from build123d import *

# Parameters (mm, degrees)
SKETCH1_W           = 60
SKETCH1_H           = 90
BOSS_EXTRUDE1_DEPTH = 3
SKETCH2_W           = 10
SKETCH2_H           = 3
SKETCH2_W_2         = 3
SKETCH2_H_2         = 10
SKETCH2_W_3         = 20
CUT_EXTRUDE2_DEPTH  = 3
SKETCH3_W           = 80
SKETCH3_H           = 120
BOSS_EXTRUDE2_DEPTH = 3
FILLET1_R           = 10
FILLET2_R           = 10
SKETCH4_R           = 1.7
CUT_EXTRUDE3_DEPTH  = 3
SKETCH5_R           = 11
CUT_EXTRUDE4_DEPTH  = 3
SKETCH6_W           = 20
SKETCH6_H           = 65
BOSS_EXTRUDE3_DEPTH = 3
FILLET3_R           = 10
SKETCH7_R           = 4
CUT_EXTRUDE5_DEPTH  = 3


with BuildPart() as part:
    # Sketch1 → Boss-Extrude1 (new body)
    with BuildSketch(Plane(origin=(0, 0, 0), x_dir=(1, 0, 0), z_dir=(0, 1, 0))):
        Rectangle(SKETCH1_W, SKETCH1_H)
    extrude(amount=BOSS_EXTRUDE1_DEPTH)

    # Sketch2 → Cut-Extrude2 (cut)
    with BuildSketch(Plane(origin=(0, 3, 0), x_dir=(1, 0, 0), z_dir=(0, 1, 0))):
        with Locations((25, 16.5)):
            Rectangle(SKETCH2_W, SKETCH2_H)
        with Locations((-28.5, 30)):
            Rectangle(SKETCH2_W_2, SKETCH2_H_2)
        with Locations((-25, 16.5)):
            Rectangle(SKETCH2_W, SKETCH2_H)
        with Locations((0, 16.5)):
            Rectangle(SKETCH2_W_3, SKETCH2_H)
        with Locations((28.5, 30)):
            Rectangle(SKETCH2_W_2, SKETCH2_H_2)
    extrude(amount=-CUT_EXTRUDE2_DEPTH, mode=Mode.SUBTRACT)

    # Sketch3 → Boss-Extrude2 (add)
    with BuildSketch(Plane(origin=(0, 3, 0), x_dir=(1, 0, 0), z_dir=(0, 1, 0))):
        Rectangle(SKETCH3_W, SKETCH3_H)
        Polygon((-30, 18), (-30, -45), (30, -45), (30, 18), (30, 25), (30, 45), (-30, 45), (-30, 35), align=None, mode=Mode.SUBTRACT)
    extrude(amount=-BOSS_EXTRUDE2_DEPTH)

    # Fillet1
    fillet1_edges = [part.edges().sort_by_distance(p)[0] for p in [
        (-40, 1.5, 60),
        (40, 1.5, 60),
    ]]
    fillet(fillet1_edges, radius=FILLET1_R)

    # Fillet2
    fillet2_edges = [part.edges().sort_by_distance(p)[0] for p in [
        (-40, 1.5, -60),
        (40, 1.5, -60),
    ]]
    fillet(fillet2_edges, radius=FILLET2_R)

    # Sketch4 → Cut-Extrude3 (cut)
    with BuildSketch(Plane(origin=(0, 3, 0), x_dir=(1, 0, 0), z_dir=(0, 1, 0))):
        with Locations(Location((15.5, -9.5, 0), (0, 0, 270))):
            Circle(SKETCH4_R)
        with Locations(Location((15.5, -40.5, 0), (0, 0, 270))):
            Circle(SKETCH4_R)
        with Locations(Location((-15.5, -40.5, 0), (0, 0, 270))):
            Circle(SKETCH4_R)
        with Locations(Location((-15.5, -9.5, 0), (0, 0, 270))):
            Circle(SKETCH4_R)
    extrude(amount=-CUT_EXTRUDE3_DEPTH, mode=Mode.SUBTRACT)

    # Sketch5 → Cut-Extrude4 (cut)
    with BuildSketch(Plane(origin=(0, 3, 0), x_dir=(1, 0, 0), z_dir=(0, 1, 0))):
        with Locations(Location((0, -25, 0), (0, 0, 270))):
            Circle(SKETCH5_R)
    extrude(amount=-CUT_EXTRUDE4_DEPTH, mode=Mode.SUBTRACT)

    # Sketch6 → Boss-Extrude3 (add)
    with BuildSketch(Plane(origin=(0, 3, 0), x_dir=(1, 0, 0), z_dir=(0, 1, 0))):
        with Locations((50, -17.5)):
            Rectangle(SKETCH6_W, SKETCH6_H)
        with Locations((-50, -17.5)):
            Rectangle(SKETCH6_W, SKETCH6_H)
    extrude(amount=-BOSS_EXTRUDE3_DEPTH)

    # Fillet3
    fillet3_edges = [part.edges().sort_by_distance(p)[0] for p in [
        (-40, 1.5, 50),
        (-60, 1.5, 50),
        (-40, 1.5, -15),
        (-60, 1.5, -15),
        (40, 1.5, -15),
        (60, 1.5, -15),
        (60, 1.5, 50),
        (40, 1.5, 50),
    ]]
    fillet(fillet3_edges, radius=FILLET3_R - 0.0001)  # a hair under: the kernel refuses the full size

    # Sketch7 → Cut-Extrude5 (cut)
    with BuildSketch(Plane(origin=(0, 3, 0), x_dir=(1, 0, 0), z_dir=(0, 1, 0))):
        with Locations(Location((-40, -15, 0), (0, 0, 270))):
            Circle(SKETCH7_R)
        with Locations(Location((40, -15, 0), (0, 0, 270))):
            Circle(SKETCH7_R)
    extrude(amount=-CUT_EXTRUDE5_DEPTH, mode=Mode.SUBTRACT)


solid = part.part
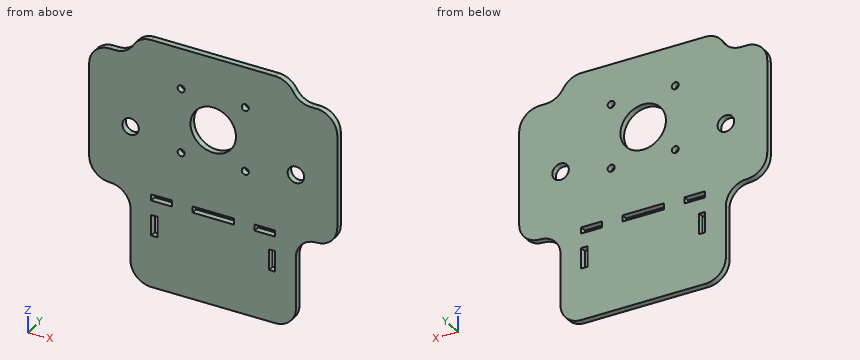
Source: CAD feature listing. Evaluate the final solid. Frame: model axes, mm. Round coordinates to 2 decimals unless told otherwise and drop trailing zeros. Loops run counter-clockwise (first coordinate to the right, second up) from the corner with the lowest first, then second, coordinate; pieces in that order, holes last.
Q1. Section B-B, the plane x = -15.5. Return loops of the section in (y, z).
Q2. Section D-D, the plane y = 0.6. State how many separate pieces and enclosed holes the cut face has, plus the area to 3 significant figures.
Q3. Section C-C, the plane z = 25. Return loops of the section in (x, y).
Q4. Ray query, line 1 (X direction, y = 1.85, z = 40.5); line 2 (X direction, y = 1.55, z = 25); line 3 (Z direction, x = 16, y = 2.6). Return the intervals inside material, ascending.
Q5. First-contact query: P1, Ø1, axis at x = 45, y = 1, coming from the +Z side; P2, Ø6.5, axis at x = 40, z = 15, coming from the -Y side; P3, Ø0.9, axis at y = 2, z = -31, coming from the +X side. Flat tips, straight axial feed; report the tip coordinate or a pass-through.
Q6. Section A-A, the plane z = 9.5. Return loops of the section in (x, y), plus the area to 3 significant figures.
Solutions:
1. outline: (0, -60) - (3, -60) - (3, 7.8) - (0, 7.8) - close; (0, 11.2) - (3, 11.2) - (3, 38.8) - (0, 38.8) - close; (0, 42.2) - (3, 42.2) - (3, 60) - (0, 60) - close
2. separate pieces: 1
2. enclosed holes: 12
2. area: 11,400 mm2
3. outline: (-60, 0) - (-11, 0) - (-11, 3) - (-60, 3) - close; (11, 0) - (60, 0) - (60, 3) - (11, 3) - close
4. line 1: x = -59.99 to -17.2, -13.8 to 13.8, 17.2 to 59.99
4. line 2: x = -60 to -11, 11 to 60
4. line 3: z = -60 to 7.88, 11.12 to 38.88, 42.12 to 60
5. P1: stops at z = 50.41
5. P2: passes through
5. P3: stops at x = 40
6. outline: (-60, 0) - (-17.2, 0) - (-17.2, 3) - (-60, 3) - close; (-13.8, 0) - (13.8, 0) - (13.8, 3) - (-13.8, 3) - close; (17.2, 0) - (60, 0) - (60, 3) - (17.2, 3) - close
6. area: 340 mm2
